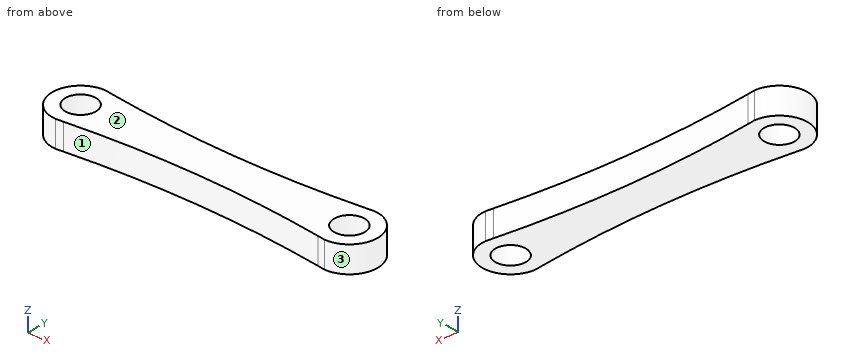
from build123d import *

# Parameters (mm, degrees)
SKETCH1_R           = 1.75
BOSS_EXTRUDE1_DEPTH = 3


with BuildPart() as part:
    # Sketch1 → Boss-Extrude1 (new body)
    with BuildSketch(Plane.XY):
        with BuildLine():
            ThreePointArc((14.688874122, 3.147153446), (0, 2.244747783), (-14.688874122, 3.147153446))
            ThreePointArc((-14.688874122, 3.147153446), (-15.094524654, 3.197885895), (-15.5, 3.25))
            ThreePointArc((-15.5, 3.25), (-18.75, 0), (-15.5, -3.25))
            ThreePointArc((-15.5, -3.25), (-15.094524654, -3.197885895), (-14.688874122, -3.147153446))
            ThreePointArc((-14.688874122, -3.147153446), (0, -2.244747783), (14.688874122, -3.147153446))
            ThreePointArc((14.688874122, -3.147153446), (15.094524654, -3.197885895), (15.5, -3.25))
            ThreePointArc((15.5, -3.25), (18.75, 0), (15.5, 3.25))
            ThreePointArc((15.5, 3.25), (15.094524654, 3.197885895), (14.688874122, 3.147153446))
        make_face()
        with Locations((-15.5, 0)):
            Circle(SKETCH1_R, mode=Mode.SUBTRACT)
        with Locations((15.5, 0)):
            Circle(SKETCH1_R, mode=Mode.SUBTRACT)
    extrude(amount=-BOSS_EXTRUDE1_DEPTH)


solid = part.part
Verification items for the finished model (mm, model axes). Face numbers are marked on the shaded views. Round coordinates to 2 decimals unless told otherwise and drop trailing zeros. Loops run counter-clockwise (first coordinate to the right, second up) from the corner with the lowest first, then second, coordinate; pieces in that order, holes last. Notation, with made-up numbers: (53, 83.5) - (81, 83.5) arc R17 cw to (81, 107.5) - close; hole circle Ø10 at (79, 38). An arc over 180 degrees is marked (long way). Use one line per item in the form item = value.
1. Scan lines: probe 1 along Y at (x, z) = (-15.5, -1.9); probe 2 along X at (y, z) = (0.25, -2.15); probe 3 along X at (y, z) = (1, -1.85). Record each from-to range of solid material in increasing order.
A:
probe_1 = -3.25 to -1.75, 1.75 to 3.25
probe_2 = -18.74 to -17.23, -13.77 to 13.77, 17.23 to 18.74
probe_3 = -18.59 to -16.94, -14.06 to 14.06, 16.94 to 18.59
2. Section check A-A on y = 0. Record the cut outline in (x, z), and give its area (3 significant figures).
A:
outline = (-18.75, -3) - (-17.25, -3) - (-17.25, 0) - (-18.75, 0) - close; (-13.75, -3) - (13.75, -3) - (13.75, 0) - (-13.75, 0) - close; (17.25, -3) - (18.75, -3) - (18.75, 0) - (17.25, 0) - close
area = 91.5 mm²
3. Section check D-D on x = 0.5. Record the cut outline in (y, z).
A:
outline = (-2.25, -3) - (2.25, -3) - (2.25, 0) - (-2.25, 0) - close
4. Section check B-B on z = -0.85. Record the cut outline in (x, y).
A:
outline = (-15.5, -3.25) arc R120 cw to (-14.69, -3.15) arc R120 cw to (14.69, -3.15) arc R120 cw to (15.5, -3.25) arc R3.25 ccw to (15.5, 3.25) arc R120 cw to (14.69, 3.15) arc R120 cw to (-14.69, 3.15) arc R120 cw to (-15.5, 3.25) arc R3.25 ccw to start; hole circle Ø3.5 at (-15.5, 0); hole circle Ø3.5 at (15.5, 0)
5. Gauge pin test, flat ends, axial feed: pin 1 Ø2 at (x, y) = (15.5, 0) entering from +Z; pin 2 Ø1 at (y, z) = (-1.5, -2.5) entering from -X; pin 3 Ø3 at (x, y) = (7, -2.5) entering from +Z. Record the tip position at first contact, or that the pin passes through.
A:
pin_1 = through
pin_2 = -18.59
pin_3 = 0
6. Section check C-C on x = 8.5. Record the cut outline in (y, z).
A:
outline = (-2.55, -3) - (2.55, -3) - (2.55, 0) - (-2.55, 0) - close
7. Draft check along X on the marked faces 1, 2 and 3. Enter one of: pulls with the +X half, pulls with the -X half, needs draft (parallel to the pull), parting line crosses it, or undercut.
A:
face_1 = undercut
face_2 = needs draft
face_3 = pulls with the +X half
